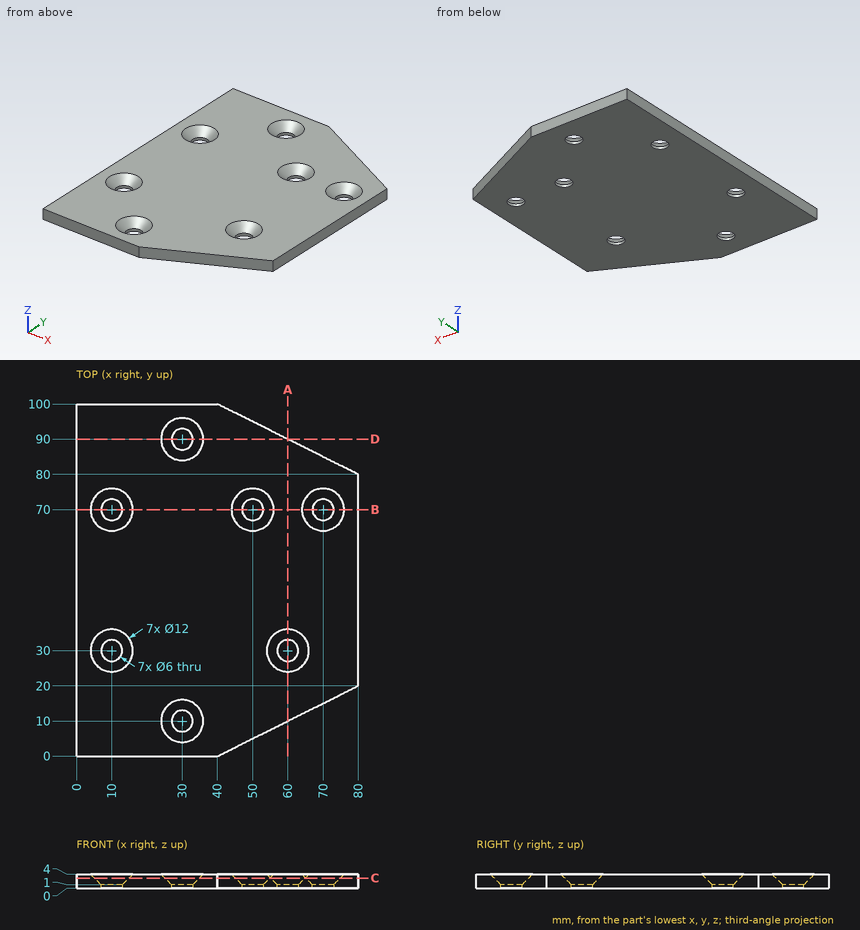
For this review, use the dimensioned drawing (mm, ordinates from the lowest corner) and the shaded views. Round coordinates to 2 decimals unless told otherwise and drop trailing zeros. Order: outer loops, then holes, each group sorted by start corner. A loop starts at its lowest first (then second) coordinate and runs counter-clockwise, first axis right, second up. Notation, with made-up numbers: (77, 52) -> (83, 52) arc R32 cw to (83, 83) -> close; hole circle Ø6 at (40.5, 86.25). An arc over 180 degrees is marked (long way). Put each result on its own line as item: value.
Q1. Add section D-D on y = 90. Write out the cut boundary in (x, z).
Check result:
outline: (0, 0) -> (27, 0) -> (27, 1) -> (24, 4) -> (0, 4) -> close; (33, 0) -> (60, 0) -> (60, 4) -> (36, 4) -> (33, 1) -> close
Q2. Add section B-B on y = 70. Write out the cut boundary in (x, z), plus the area to 3 significant figures.
Check result:
outline: (0, 0) -> (7, 0) -> (7, 1) -> (4, 4) -> (0, 4) -> close; (13, 0) -> (47, 0) -> (47, 1) -> (44, 4) -> (16, 4) -> (13, 1) -> close; (53, 0) -> (67, 0) -> (67, 1) -> (64, 4) -> (56, 4) -> (53, 1) -> close; (73, 0) -> (80, 0) -> (80, 4) -> (76, 4) -> (73, 1) -> close
area: 221 mm2
Q3. Insertion check: pin 1 Ø8 at (x, y) = (10, 70) entering from -Z. The pin has a flat end and moves straight along its axis. Give the tip position at first contact, or say it passes through.
Check result:
pin 1: z = 0
Q4. Add section A-A on x = 60. Write out the cut boundary in (y, z), plus the area to 3 significant figures.
Check result:
outline: (10, 0) -> (27, 0) -> (27, 1) -> (24, 4) -> (10, 4) -> close; (33, 0) -> (90, 0) -> (90, 4) -> (36, 4) -> (33, 1) -> close
area: 287 mm2
Q5. Add section C-C on z = 2.9. Write out the cut boundary in (x, y), plus the area to 3 significant figures.
Check result:
outline: (0, 0) -> (40, 0) -> (80, 20) -> (80, 80) -> (40, 100) -> (0, 100) -> close; hole circle Ø9.8 at (10, 30); hole circle Ø9.8 at (10, 70); hole circle Ø9.8 at (30, 10); hole circle Ø9.8 at (30, 90); hole circle Ø9.8 at (50, 70); hole circle Ø9.8 at (60, 30); hole circle Ø9.8 at (70, 70)
area: 6,670 mm2
Q6. For probe 1 along Y at (x, z) = (14, 3.25); probe 2 along Y at (x, z) = (26.5, 2.2); probe 3 along Y at (x, z) = (62, 2.7), list the stretches that pass through material, from the lowest coordinate up. Write a range as [from, to].
Check result:
probe 1: [0, 26.6], [33.4, 66.6], [73.4, 100]
probe 2: [0, 7.68], [12.32, 87.68], [92.32, 100]
probe 3: [11, 25.75], [34.25, 89]
